```python
from build123d import *

# Parameters (mm, degrees)
F0_W      = 609.6
F0_H      = 101.6
F1_DEPTH  = 3.175
F2_R      = 7.14375
F3_DEPTH  = 3.176
F4_R      = 26.9875
F5_DEPTH  = 3.176
F6_R      = 20.32
F7_DEPTH  = 3.176
F8_R      = 7.9375
F9_DEPTH  = 3.176
F10_R     = 3.175
F11_DEPTH = 3.176


# Not quite as in the source:
# - a feature names something its author has since deleted; it is built from what else it names


with BuildPart() as f1:
    # F0 (on Front) → F1 (new body)
    with BuildSketch(Plane.XZ):
        with Locations((304.8, 50.8)):
            Rectangle(F0_W, F0_H)
    extrude(amount=F1_DEPTH)

    # F2 (on face) → F3 (cut, through all)
    with BuildSketch(Plane.XZ.offset(3.175)):
        with Locations((31.75, 31.75)):
            Circle(F2_R)
        with Locations((88.9, 31.75)):
            Circle(F2_R)
        with Locations((146.05, 31.75)):
            Circle(F2_R)
        with Locations((203.2, 31.75)):
            Circle(F2_R)
        with Locations((260.35, 31.75)):
            Circle(F2_R)
        with Locations((317.5, 31.75)):
            Circle(F2_R)
        with Locations((374.65, 31.75)):
            Circle(F2_R)
        with Locations((431.8, 31.75)):
            Circle(F2_R)
    extrude(amount=-F3_DEPTH, mode=Mode.SUBTRACT)

    # F4 (on face) → F5 (cut, through all)
    with BuildSketch(Plane.XZ.offset(3.175)):
        with Locations((501.65, 50.8)):
            Circle(F4_R)
    extrude(amount=-F5_DEPTH, mode=Mode.SUBTRACT)

    # F6 (on face) → F7 (cut, through all)
    with BuildSketch(Plane.XZ.offset(3.175)):
        with Locations((571.5, 50.8)):
            Circle(F6_R)
    extrude(amount=-F7_DEPTH, mode=Mode.SUBTRACT)

    # F8 (on face) → F9 (cut, through all)
    with BuildSketch(Plane.XZ.offset(3.175)):
        with Locations((31.75, 66.675)):
            Circle(F8_R)
        with Locations((88.9, 66.675)):
            Circle(F8_R)
        with Locations((146.05, 66.675)):
            Circle(F8_R)
        with Locations((203.2, 66.675)):
            Circle(F8_R)
        with Locations((260.35, 66.675)):
            Circle(F8_R)
        with Locations((317.5, 66.675)):
            Circle(F8_R)
        with Locations((374.65, 66.675)):
            Circle(F8_R)
        with Locations((431.8, 66.675)):
            Circle(F8_R)
    extrude(amount=-F9_DEPTH, mode=Mode.SUBTRACT)

    # F10 (on face) → F11 (cut, through all)
    with BuildSketch(Plane.XZ.offset(3.175)):
        with Locations((63.5, 92.075)):
            Circle(F10_R)
        with Locations((304.8, 92.075)):
            Circle(F10_R)
        with Locations((546.1, 92.075)):
            Circle(F10_R)
    extrude(amount=-F11_DEPTH, mode=Mode.SUBTRACT)


solid = f1.part
```
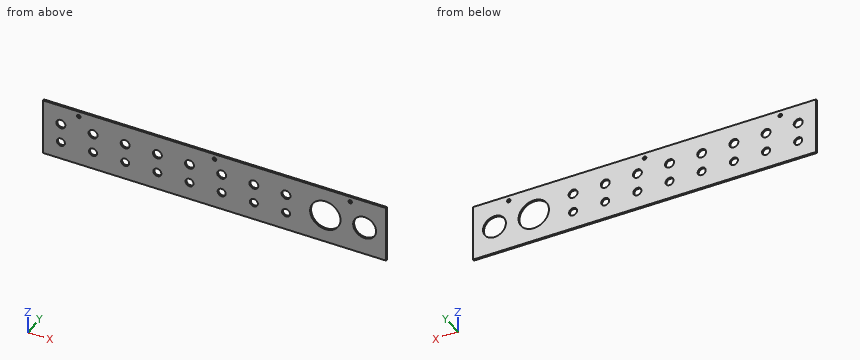
CAD build for the part. Positions are in the model's coordinates, mm. Round coordinates to 2 decimals unless told otherwise and drop trailing zeros. Order: outer loops, then holes, each group sorted by start corner. A loop starts at its lowest first (then second) coordinate and runs counter-clockwise, first axis right, second up. Notation, with made-up numbers: (-34.5, -23.75) - (15.5, -23.75) arc R16 cw to (15.5, -5.75) - close; hole circle Ø6 at (68.5, -3). An arc over 180 degrees is marked (long way). Answer as CSV lines item,"result". Start each with the question number.
1. Saw through at D-D, the plane y = -2.65. Count the separate pieces of the cut face and the enclosed holes in it, and give its area (3 significant figures).
2. Pin check, flat tip, straight feed: pin 1 (4 mm diameter, centred on x = 304.8, z = 92.075, fed in from -Y). Stop position of the tip, or through.
3. Saw through at C-C, the plane z = 44. Write the cut outline in (x, y) (3 decimals).
4. Saw through at B-B, the plane x = 374.65. Write the cut outline in (y, z) (1 decimal).
5. Saw through at A-A, the plane x = 571.5. Write the cut outline in (y, z) (3 decimals), and give its area (3 significant figures).
6. Drill centre lines: L1, parallel to X at y = -0.5, z = 91.5; L2, parallel to X at y = -0.5, z = 53; L3, parallel to Z at x = 31.75, y = -1.4. Where is each one in solid material? Low to high. Write a range as [from, to].
Model answer:
1,separate pieces,"1"
1,enclosed holes,"21"
1,area,"55,400 mm²"
2,pin 1,"passes through"
3,outline,"(0, -3.175) - (475.533, -3.175) - (475.533, 0) - (0, 0) - close; (527.767, -3.175) - (552.352, -3.175) - (552.352, 0) - (527.767, 0) - close; (590.648, -3.175) - (609.6, -3.175) - (609.6, 0) - (590.648, 0) - close"
4,outline,"(-3.2, 0) - (0, 0) - (0, 24.6) - (-3.2, 24.6) - close; (-3.2, 38.9) - (0, 38.9) - (0, 58.7) - (-3.2, 58.7) - close; (-3.2, 74.6) - (0, 74.6) - (0, 101.6) - (-3.2, 101.6) - close"
5,outline,"(-3.175, 0) - (0, 0) - (0, 30.48) - (-3.175, 30.48) - close; (-3.175, 71.12) - (0, 71.12) - (0, 101.6) - (-3.175, 101.6) - close"
5,area,"194 mm²"
6,L1,"x = [0, 60.38], [66.62, 301.68], [307.92, 542.98], [549.22, 609.6]"
6,L2,"x = [0, 474.75], [528.55, 551.3], [591.7, 609.6]"
6,L3,"z = [0, 24.61], [38.89, 58.74], [74.61, 101.6]"
